Geometry: final body of the model. Coordinates: model frame, mm. A direction names the side the tool comes from. Round coordinates to 2 decimals unless told otherwise and drop trailing zeros. Loops run counter-clockwise (first coordinate to the right, second up) from the corner with the lowest first, then second, coordinate; pieces in that order, holes last. Notation, with made-up numbers: (62.5, 9) - (96.5, 9) arc R28 ccw to (96.5, 35) - close; hole circle Ø6 at (-5, 54.25). An arc over 180 degrees is marked (long way). Use CSV: the item, a comma, the result in double quotes.
from build123d import *

# Parameters (mm, degrees)
SKETCH1_W           = 15
SKETCH1_H           = 45
BOSS_EXTRUDE1_DEPTH = 10
SKETCH4_W           = 15
SKETCH4_H           = 6.8
CUT_EXTRUDE2_DEPTH  = 41.8
SKETCH5_R           = 1
CUT_EXTRUDE3_DEPTH  = 47.703854231
SKETCH6_R           = 1
SKETCH6_W           = 11.6
SKETCH6_H           = 22.1
CUT_EXTRUDE4_DEPTH  = 25.67265693


with BuildPart() as part:
    # Sketch1 → Boss-Extrude1 (new body)
    with BuildSketch(Plane(origin=(0, 0, 0), x_dir=(1, 0, 0), z_dir=(0, 1, 0))):
        Rectangle(SKETCH1_W, SKETCH1_H)
    extrude(amount=BOSS_EXTRUDE1_DEPTH)

    # Sketch4 → Cut-Extrude2 (cut)
    with BuildSketch(Plane(origin=(0, 0, -22.5), x_dir=(-1, 0, 0), z_dir=(0, 0, -1))):
        with Locations((0, 6.6)):
            Rectangle(SKETCH4_W, SKETCH4_H)
    extrude(amount=-CUT_EXTRUDE2_DEPTH, mode=Mode.SUBTRACT)

    # Sketch5 → Cut-Extrude3 (cut, through all)
    with BuildSketch(Plane.XY.offset(22.5)):
        with Locations((-2, 7)):
            Circle(SKETCH5_R)
        with Locations((2, 7)):
            Circle(SKETCH5_R)
    extrude(amount=-CUT_EXTRUDE3_DEPTH, mode=Mode.SUBTRACT)

    # Sketch6 → Cut-Extrude4 (cut, through all)
    with BuildSketch(Plane(origin=(0, 3.2, 0), x_dir=(1, 0, 0), z_dir=(0, 1, 0))):
        with Locations(Location((0, -8.8, 0), (0, 0, 270))):
            Circle(SKETCH6_R)
        with Locations(Location((0, 17.91, 0), (0, 0, 270))):
            Circle(SKETCH6_R)
        with Locations((0, 4.45)):
            Rectangle(SKETCH6_W, SKETCH6_H)
    extrude(amount=-CUT_EXTRUDE4_DEPTH, mode=Mode.SUBTRACT)


solid = part.part
Item 1: Reachability of faces 1 (the flat face through (-5.8, 2, -4)), 2 (the flat face through (0, 7, 19.3)), 3 (the flat face through (2, 0, 10)) from +Z, -Z, +X, -X, +Y, -Y: full face, straight path, thin tool, end or side. Return the list, or none.
Final values:
face 1,"+Y, -Y"
face 2,"-Z, +X, -X, +Y"
face 3,"+Z, -Z, +X, -X, -Y"
Item 2: Section D-D on x = 2. Return the cut outline in (y, z), plus the area to 3 significant figures.
Final values:
outline,"(0, -22.5) - (3.2, -22.5) - (3.2, -15.5) - (0, -15.5) - close; (0, 6.6) - (3.2, 6.6) - (3.2, 19.3) - (6, 19.3) - (6, 22.5) - (0, 22.5) - close; (8, 19.3) - (10, 19.3) - (10, 22.5) - (8, 22.5) - close"
area,"88.6 mm²"
Item 3: Section C-C on x = 0. Return the cut outline in (y, z), plus the area to 3 significant figures.
Final values:
outline,"(0, -22.5) - (3.2, -22.5) - (3.2, -18.91) - (0, -18.91) - close; (0, -16.91) - (3.2, -16.91) - (3.2, -15.5) - (0, -15.5) - close; (0, 6.6) - (3.2, 6.6) - (3.2, 7.8) - (0, 7.8) - close; (0, 9.8) - (3.2, 9.8) - (3.2, 19.3) - (10, 19.3) - (10, 22.5) - (0, 22.5) - close"
area,"82.2 mm²"
Item 4: Material intervals for line 1 (Z direction, x = 3.25, y = 2.5); line 2 (Y direction, x = -2, z = 20.05); line 3 (X direction, y = 2.3, z = 8.8), sorted ascending.
Final values:
line 1,"z = -22.5 to -15.5, 6.6 to 22.5"
line 2,"y = 0 to 6, 8 to 10"
line 3,"x = -7.5 to -1, 1 to 7.5"
Item 5: Mould query, pull axis X, two halves, no side actions, for faces 4 (the flat face through (-7.5, 3, 5)), 5 (the cylindrical face through (2, 8, 21)), 6 (the flat face through (7, 3.2, -2)), 7 (the flat face through (0, 2, 6.6)). Classes: released by +X, released by -X, zero draft, split by the parting line, or undercut.
Final values:
face 4,"released by -X"
face 5,"undercut"
face 6,"zero draft"
face 7,"undercut"
Item 6: Section A-A on x = 4.75. Return the cut outline in (y, z).
Final values:
outline,"(0, -22.5) - (3.2, -22.5) - (3.2, -15.5) - (0, -15.5) - close; (0, 6.6) - (3.2, 6.6) - (3.2, 19.3) - (10, 19.3) - (10, 22.5) - (0, 22.5) - close"
Item 7: Pin query (flat end, axial travel): P1, Ø4, axis at x = -5.5, z = 1, coming from the +Y side; P2, Ø2, axis at x = 2, y = 7.5, coming from the -Z side; P3, Ø1.6, axis at x = -2, y = 7, coming from the -Z side. Return the tip coordinate at first contact, or that it passes through.
Final values:
P1,"stops at y = 3.2"
P2,"stops at z = 19.3"
P3,"passes through"
Item 8: Section B-B on z = -0.5. Return the cut outline in (x, y), plus the area to 3 significant figures.
Final values:
outline,"(-7.5, 0) - (-5.8, 0) - (-5.8, 3.2) - (-7.5, 3.2) - close; (5.8, 0) - (7.5, 0) - (7.5, 3.2) - (5.8, 3.2) - close"
area,"10.9 mm²"
